from build123d import *

# Parameters (mm, degrees)
BASENUT_START = -3.8
BASENUTSKE_R  = 1.65
BASENUT_DEPTH = 3.8
SCALA1_SCALE  = 1.05


# Read off the part's stored shape, not the designer's step: ThreadSchematic
with BuildPart() as part:
    # BaseNutSke → BaseNut (new body)
    with BuildSketch(Plane.XY.offset(BASENUT_START)):
        Polygon((3.5, 2.020725942), (3.5, -2.020725942), (0, -4.041451884), (-3.5, -2.020725942), (-3.5, 2.020725942), (0, 4.041451884), align=None)
        Circle(BASENUTSKE_R, mode=Mode.SUBTRACT)
    extrude(amount=BASENUT_DEPTH)

    # Sketch5 (on Front Plane) → EndChamfer (revolve, cut)
    with BuildSketch(Plane.XY):
        Polygon((3.7746, 2), (3.505020098, 1.615), (3.8254, 1.615), (3.8254, 2), align=None)
    revolve(axis=Axis((3.7746, 2, 0), (-0.5735764363510472, -0.8191520442889912, 0)), mode=Mode.SUBTRACT)

    # Sketch3 → Double-Chamfer (revolve, cut)
    with BuildSketch(Plane(origin=(0, 0, 0), x_dir=(0, 0, -1), z_dir=(1, 0, 0))):
        Polygon((3.8, 3.5), (3.487392609, 4.041451884), (3.487392609, 14.041451884), (13.8, 14.041451884), (13.8, 3.5), align=None)
        Polygon((0.312607391, 14.041451884), (-10, 14.041451884), (-10, 3.5), (0, 3.5), (0.312607391, 4.041451884), align=None)
    revolve(axis=Axis((0, 0, 0), (0, 0, -1)), mode=Mode.SUBTRACT)

    # ThreadSchematic outline → ThreadSchematic (revolve, cut)
    with BuildSketch(Plane.XZ):
        Polygon((1.65, 0), (1.65, -0.245072638), (2, 0), align=None)
        Polygon((2, -3.7746), (1.65, -3.529527362), (1.65, -3.8), (2, -3.8), align=None)
    revolve(axis=Axis((0, 0, 0), (0, 0, 1)), mode=Mode.SUBTRACT)


with BuildPart() as part_1:
    # Scala1: scaled about (0, 0, -1.898579805)
    add(part.part.scale(SCALA1_SCALE).moved(Location((0, 0, 0.09492899))))


solid = part_1.part
Geometry: final body of the model. Coordinates: model frame, mm. Give positions to 0.01 mm unless a question says otherwise; leave off trailing zeros. Write each loop counter-clockwise with the first axis right and the second up, starting at its lowest first coordinate (ties: lowest second). Pieces come first, ordered by that corner, then holes.
(1) Ray query, line 1 (Y direction, x = 1, z = -1.6); line 2 (X direction, y = -0.5, z = -1) (3 decimals); line 3 (X direction, y = 2.25, z = -2.1). Return the intervals inside material, ascending.
(2) Mould query, pull axis X, two halves, no side actions, for faces 1 (the cylindrical face through (0.93, 1.46, -1.91)), 2 (the flat face through (-3.675, 0, -2)), 3 (the conical face through (-0.009, 3.813, 0.015)), 4 (the conical face through (3.298, 1.915, -3.815)). Classes: released by +X, released by -X, zero draft, split by the parting line, or undercut.
(3) First-contact query: P1, Ø4, axis at x = 0, y = 0, coming from the +Z side; P2, Ø2, axis at x = -2.5, z = -1, coming from the +Y side; P3, Ø1.5, axis at x = 1.5, z = -2.5, coming from the +Y side. Flat tips, straight axial feed; report the tip coordinate or a pass-through.
(4) Cut plane A-A, the plane z = -1.8. Return loops of the section in (x, y) (1 decimal), then the cut area to 3 significant figures.
Values follow:
1. line 1: y = -3.67 to -1.41, 1.41 to 3.67
1. line 2: x = -3.675 to -1.659, 1.659 to 3.675
1. line 3: x = -3.45 to 3.45
2. face 1: undercut
2. face 2: released by -X
2. face 3: split by the parting line
2. face 4: released by +X
3. P1: stops at z = 0.02
3. P2: stops at y = 3.38
3. P3: stops at y = 3.81
4. outline: (-3.7, -2.1) - (0, -4.2) - (3.7, -2.1) - (3.7, 2.1) - (0, 4.2) - (-3.7, 2.1) - close; hole circle Ø3.5 at (0, 0)
4. area: 37.4 mm2
